Design review of the part built by this model. Coordinates are the model's own, in mm. A direction names the side the tool comes from. Coordinates: 2 decimals unless noted, no trailing zeros. Write each loop counter-clockwise with the first axis right and the second up, starting at its lowest first coordinate (ties: lowest second). Pieces come first, ordered by that corner, then holes.
Q1. To check wall thickness, follow probe 1 along Y at (x, z) = (-6, 574); probe 2 along Y at (x, z) = (-0.5, 1272); probe 3 along X at (y, z) = (0, 556). State the ranges of each line that lie inside material, in increasing order.
Q2. The part is to be moulded in two halves that separate along X. For faces 1 (the face through (296.49, 95.37, 691.23)), 2 (the face through (42.17, 316.1, 1520.3)), 3 (the face through (-266.959, -244.795, 73.116)), 4 (the face through (326, 2, 1746)), say which applies: +X half, -X half, draft (parallel to the pull), parting line (faces both ways), or undercut.
Q3. Add section A-A, the plane x = 0. Give the boundary of the cut face in (y, z).
Q4. Machinability: for faces 5 (the face through (336, -139, 50.8)), 6 (the face through (309, -55, 0)), which of the approach directions +Z, -Z, +X, -X, +Y, -Y give a long, thin tool a straight path to every point of the face, cutting with its end or side? Answer none if there is none.
Q5. Add section C-C, the plane z = 1531.5. Give the boundary of the cut face in (x, y), plus the area to 3 significant figures.
Q6. Add section B-B, the plane z = 720.5. Give the boundary of the cut face in (x, y), plus the area to 3 significant figures.
Q7. Clearance check with flat-ended pins moving along their axes: pin 1 Ø5 at (y, z) = (-227, 563.5) entering from +X; pin 2 Ø3 at (x, z) = (-6, 801) entering from +Y; pin 3 Ø1.5 at (x, z) = (149.5, 1324) entering from +Y. State where each tip first meets the part, or that it passes through.
Autodesk Inventor part; units mm, degrees
ref_plane "YZ Plane" through (0, 0, 0) normal (1, 0, 0) x (0, 1, 0)
ref_plane "XZ Plane" through (0, 0, 0) normal (0, 1, 0) x (-1, 0, 0)
ref_plane "XY Plane" through (0, 0, 0) normal (0, 0, 1) x (1, 0, 0)
sketch "Sketch1" plane through (0, 0, 0) normal (0, 0, 1) x (1, 0, 0)
  circle A0 centre (0, 0) radius 381.254
  dimension "d0" = 762.508
extrude "Extrusion1" add sketch "Sketch1" along normal blind 50.8
sketch "Sketch2" plane through (0, 0, 0) normal (0, 0, 1) x (1, 0, 0)
  circle A0 centre (0, 0) radius 362.204
  dimension "d3" = 724.408
extrude "Extrusion2" add sketch "Sketch2" along normal blind 95.25
sketch "Sketch3" plane through (0, 0, 0) normal (0, 0, 1) x (1, 0, 0)
  circle A0 centre (0, 0) radius 349.25
  dimension "d6" = 698.5
extrude "Extrusion3" add sketch "Sketch3" along normal blind 1746
sketch "Sketch4" plane through (0, 0, 1746) normal (0, 0, 1) x (1, 0, 0)
  circle A0 centre (-6.35, 0) radius 317.5
  point P0 (0, 0)
  dimension "d9" = 635
  dimension "d24" = 6.35
extrude "Extrusion4" cut sketch "Sketch4" against normal through all
chamfer "Chamfer1" distance 0.7937 angle 45 1 edges at (-381.254, 0, 50.8)
fillet "Fillet1" radius 0.7937 1 edges at (-362.204, 0, 50.8)
fillet "Fillet2" radius 0.7937 1 edges at (-349.25, 0, 95.25)
sketch "Sketch5" plane through (0, 0, 0) normal (0, 1, 0) x (-1, 0, 0)
  line L0 (-311.15, 1746) -> (323.85, 1746)
  line L1 (-311.15, 1746) -> (323.85, 1213.1717)
  line L2 (323.85, 1213.1717) -> (349.25, 1213.1717)
  line L3 (349.25, 1213.1717) -> (349.25, 1746)
  line L4 (349.25, 1746) -> (323.85, 1746)
  line L5 (349.25, 96.0438) -> (349.25, 1746) construction
  point P0 (0, 0)
  dimension "d18" = 40
extrude "Extrusion5" cut sketch "Sketch5" along normal through all both and the other way through all
equation "\"BendRadius\" = Thickness"
equation "\"BendReliefWidth\" = Thickness"
equation "\"BendReliefDepth\" = 0.5 * Thickness"
equation "\"CornerReliefSize\" = 4 * Thickness"
equation "\"MinimumRemnant\" = 2 * Thickness"
equation "\"TransitionRadius\" = BendRadius"
equation "\"JacobiRadiusSize\" = Thickness"
equation "\"GapSize\" = Thickness"
properties part number "A1-19010-100-02 HCWI nozzle insert" material "Iron, Cast"
Here are the results:
1. probe 1: y = -349.2 to -317.5, 317.5 to 349.2
1. probe 2: y = -349.25 to -317.45, 317.45 to 349.25
1. probe 3: x = -349.25 to -323.85, 311.15 to 349.25
2. face 1: undercut
2. face 2: -X half
2. face 3: parting line
2. face 4: draft
3. outline: (-381.25, 0) - (-317.44, 0) - (-317.44, 1484.91) - (-349.25, 1484.91) - (-349.25, 96.04) arc R0.79 cw to (-350.04, 95.25) - (-362.2, 95.25) - (-362.2, 51.59) arc R0.79 cw to (-363, 50.8) - (-380.46, 50.8) - (-381.25, 50.01) - close; (317.44, 0) - (381.25, 0) - (381.25, 50.01) - (380.46, 50.8) - (363, 50.8) arc R0.79 cw to (362.2, 51.59) - (362.2, 95.25) - (350.04, 95.25) arc R0.79 cw to (349.25, 96.04) - (349.25, 1484.91) - (317.44, 1484.91) - close
4. face 5: +Z
4. face 6: -Z, +X, -X, +Y, -Y
5. outline: (55.52, -344.81) arc R349.25 ccw to (55.52, 344.81) - (55.52, 311.41) arc R317.5 cw to (55.52, -311.41) - close
5. area: 33,700 mm2
6. outline: circle Ø698.5 at (0, 0); hole circle Ø635 at (-6.35, 0)
6. area: 66,500 mm2
7. pin 1: stops at x = 267.54
7. pin 2: stops at y = 349.22
7. pin 3: stops at y = 315.99
